Geometry check sheet. Reference: the model listing, model coordinates, mm. A direction names the side the tool comes from. Give positions to 0.01 mm unless a question says otherwise; leave off trailing zeros. Write each loop counter-clockwise with the first axis right and the second up, starting at its lowest first coordinate (ties: lowest second). Pieces come first, ordered by that corner, then holes. Notation, with made-up numbers: M -3.75,23.5 L 2.25,23.5 A21 cw 2.25,47.5 Z; hole C 48.25,-21 d11. An arc over 180 degrees is marked long. Write each question's results on one line, items separated by ' | '.
```python
from build123d import *

# Parameters (mm, degrees)
BOSS_EXTRUDE1_DEPTH = 10
FILLET2_R           = 7


with BuildPart() as part:
    # Sketch1 → Boss-Extrude1 (new body)
    with BuildSketch(Plane(origin=(0, 0, 0), x_dir=(1, 0, 0), z_dir=(0, 1, 0))):
        with BuildLine():
            Line((0, 0), (0, 180))
            Line((0, 180), (-24.84953376, 180))
            Line((-24.84953376, 180), (-24.84953376, 241.105739003))
            Line((-24.84953376, 241.105739003), (-9.081721857, 241.105739003))
            Line((-9.081721857, 241.105739003), (-9.081721857, 193.469393381))
            Line((-9.081721857, 193.469393381), (-6.872448555, 193.469393381))
            Line((-6.872448555, 193.469393381), (-6.872448555, 241.105739003))
            Line((-6.872448555, 241.105739003), (8.895363349, 241.105739003))
            Line((8.895363349, 241.105739003), (8.895363349, 193.469393381))
            Line((8.895363349, 193.469393381), (11.104636651, 193.469393381))
            Line((11.104636651, 193.469393381), (11.104636651, 241.105739003))
            Line((11.104636651, 241.105739003), (26.872448555, 241.105739003))
            Line((26.872448555, 241.105739003), (26.872448555, 193.469393381))
            Line((26.872448555, 193.469393381), (29.081721857, 193.469393381))
            Line((29.081721857, 193.469393381), (29.081721857, 241.105739003))
            Line((29.081721857, 241.105739003), (44.84953376, 241.105739003))
            Line((44.84953376, 241.105739003), (44.84953376, 180))
            Line((44.84953376, 180), (20, 180))
            Line((20, 180), (20, 0))
            ThreePointArc((20, 0), (10, -10), (0, 0))
        make_face()
    extrude(amount=BOSS_EXTRUDE1_DEPTH)

    # Fillet2
    fillet2_edges = [part.edges().sort_by_distance(p)[0] for p in [
        (0, 5, -180),
        (-24.84953376, 5, -180),
        (44.84953376, 5, -180),
        (20, 5, -180),
    ]]
    fillet(fillet2_edges, radius=FILLET2_R)


solid = part.part
```
Q1. Section check B-B (z = -6). Enter the section's corners in (x, y), then the cut area to 3 significant figures.
Answer key:
outline: M 0,0 L 20,0 L 20,10 L 0,10 Z | area: 200 mm2
Q2. Depth check by flat-ended pin: P1, Ø1, axis at y = 6.5, z = -45.5, coming from the +X side; P2, Ø2, axis at x = -9, y = 7, coming from the +Z side; P3, Ø6, axis at x = 29, z = -175, coming from the +Y side; P4, Ø0.7, axis at x = 27.5, y = 6, coming from the -Z side. Enter the tip coordinate at first touch or a pass-through.
Answer key:
P1: stops at x = 20 | P2: stops at z = -180 | P3: passes through | P4: stops at z = -193.47
Q3. Section check C-C (x = 40). Enter the section's corners in (y, z).
Answer key:
outline: M 0,-241.11 L 10,-241.11 L 10,-180.34 L 0,-180.34 Z
Q4. Release check for a two-part mould opening along X. For faces 4 (the face through (10, 5, 10)), 5 (the face through (-24.85, 5, -214)), 6 (the face through (-12, 5, -180)), 7 (the face through (29.082, 5, -217)) record: released by +X, released by -X, zero draft, split by the parting line, or undercut.
Answer key:
face 4: split by the parting line | face 5: released by -X | face 6: zero draft | face 7: undercut
Q5. Section check A-A (y = 3). Enter the section's corners in (x, z), then the cut area to 3 significant figures.
Answer key:
outline: M -24.85,-241.11 L -9.08,-241.11 L -9.08,-193.47 L -6.87,-193.47 L -6.87,-241.11 L 8.9,-241.11 L 8.9,-193.47 L 11.1,-193.47 L 11.1,-241.11 L 26.87,-241.11 L 26.87,-193.47 L 29.08,-193.47 L 29.08,-241.11 L 44.85,-241.11 L 44.85,-187 A7 ccw 37.85,-180 L 27,-180 A7 cw 20,-173 L 20,0 A10 ccw 0,0 L 0,-173 A7 cw -7,-180 L -17.85,-180 A7 ccw -24.85,-187 Z | area: 7,700 mm2
Q6. Access from +Z, -Z, +X, -X, +Y, -Y to the whole of each face (thin tool, end or side, straight path). Record for faces 1 (the face through (0, 5, -85)), 2 (the face through (33, 5, -180)), 3 (the face through (8.895, 5, -218)).
Answer key:
face 1: +Z, -X, +Y, -Y | face 2: +Z, +X, +Y, -Y | face 3: -Z, +Y, -Y
Q7. Material ranges on probe 1 along X at (y, z) = (5, -229); probe 2 along Z at (x, y) = (28, 5.5); probe 3 along X at (y, z) = (6.75, -93), recorded low to high. Write a range as [from, to].
Answer key:
probe 1: x = [-24.85, -9.08], [-6.87, 8.9], [11.1, 26.87], [29.08, 44.85] | probe 2: z = [-193.47, -180] | probe 3: x = [0, 20]
